```python
from build123d import *

# Parameters (mm, degrees)
SKETCH_1_W          = 10
SKETCH_1_H          = 5
EXTRUDE_1_DEPTH     = 0.5
SKETCH_2_W          = 3
SKETCH_2_H          = 3
EXTRUDE_2_DEPTH     = 0.5
SKETCH_3_W          = 10
SKETCH_3_H          = 5
EXTRUDE_3_DEPTH     = 0.5
EXTRUDE_4_DEPTH     = 5
CUT_EXTRUDE_3_DEPTH = 5
SKETCH_6_W          = 1.6
SKETCH_6_H          = 1.6
CUT_EXTRUDE_4_DEPTH = 1.5
SKETCH_7_W          = 10
SKETCH_7_H          = 0.5
CUT_EXTRUDE_5_DEPTH = 1
SKETCH_8_W          = 10
SKETCH_8_H          = 4
EXTRUDE_5_DEPTH     = 1
SKETCH_11_W         = 10
SKETCH_11_H         = 4
SKETCH_11_W_2       = 3
SKETCH_11_H_2       = 3
CUT_EXTRUDE_6_DEPTH = 0.5
CUT_EXTRUDE_7_REACH = 8.124
SKETCH_6_2_W        = 1.6
SKETCH_6_2_H        = 1.6
SKETCH_12_W         = 10
SKETCH_12_H         = 5
CUT_EXTRUDE_8_DEPTH = 6.937171044
SKETCH_13_W         = 3
SKETCH_13_H         = 3
EXTRUDE_6_DEPTH     = 3
SKETCH_14_W         = 1.7
SKETCH_14_H         = 1.7
CUT_EXTRUDE_9_DEPTH = 4


with BuildPart() as part:
    # 草图1 → 凸台-拉伸1 (new body)
    with BuildSketch(Plane(origin=(0, 0, 0), x_dir=(1, 0, 0), z_dir=(0, 1, 0))):
        Rectangle(SKETCH_1_W, SKETCH_1_H)
    extrude(amount=EXTRUDE_1_DEPTH)

    # 草图2 → 凸台-拉伸2 (add)
    with BuildSketch(Plane(origin=(0, 0.5, 0), x_dir=(1, 0, 0), z_dir=(0, 1, 0))):
        Rectangle(SKETCH_2_W, SKETCH_2_H)
    extrude(amount=EXTRUDE_2_DEPTH)

    # 草图3 → 凸台-拉伸3 (add)
    with BuildSketch(Plane(origin=(0, 1, 0), x_dir=(1, 0, 0), z_dir=(0, 1, 0))):
        Rectangle(SKETCH_3_W, SKETCH_3_H)
    extrude(amount=EXTRUDE_3_DEPTH)

    # 草图4 → 凸台-拉伸4 (add)
    with BuildSketch(Plane.XY.offset(2.5)):
        with BuildLine():
            Line((-5, 1.5), (5, 1.5))
            ThreePointArc((5, 1.5), (0, 2.5), (-5, 1.5))
        make_face()
    extrude(amount=-EXTRUDE_4_DEPTH)

    # 草图5 → 切除-拉伸3 (cut)
    with BuildSketch(Plane.XY.offset(2.5)):
        with BuildLine():
            Line((-4.75, 2.75), (-4.25, 2.75))
            Line((-4.25, 2.75), (-4.25, 1.535662375))
            ThreePointArc((-4.25, 1.535662375), (-4.50094573, 1.445961936), (-4.75, 1.35113631))
            Line((-4.75, 1.35113631), (-4.75, 2.75))
        make_face()
        with BuildLine():
            Line((-3.75, 2.75), (-3.75, 1.697389285))
            ThreePointArc((-3.75, 1.697389285), (-3.500697998, 1.769788877), (-3.25, 1.837195875))
            Line((-3.25, 1.837195875), (-3.25, 2.75))
            Line((-3.25, 2.75), (-3.75, 2.75))
        make_face()
        with BuildLine():
            Line((-2.75, 2.75), (-2.75, 1.95580576))
            ThreePointArc((-2.75, 1.95580576), (-2.500480176, 2.007256715), (-2.25, 2.053808027))
            Line((-2.25, 2.053808027), (-2.25, 2.75))
            Line((-2.25, 2.75), (-2.75, 2.75))
        make_face()
        with BuildLine():
            Line((-1.75, 2.75), (-1.75, 2.131673028))
            ThreePointArc((-1.75, 2.131673028), (-1.50028119, 2.163138904), (-1.25, 2.189764295))
            Line((-1.25, 2.189764295), (-1.25, 2.75))
            Line((-1.25, 2.75), (-1.75, 2.75))
        make_face()
        with BuildLine():
            Line((-0.75, 2.75), (-0.75, 2.228347352))
            ThreePointArc((-0.75, 2.228347352), (-0.500092618, 2.240377492), (-0.25, 2.247595932))
            Line((-0.25, 2.247595932), (-0.25, 2.75))
            Line((-0.25, 2.75), (-0.75, 2.75))
        make_face()
        with BuildLine():
            Line((0.25, 2.75), (0.25, 2.247595932))
            ThreePointArc((0.25, 2.247595932), (0.500092618, 2.240377492), (0.75, 2.228347352))
            Line((0.75, 2.228347352), (0.75, 2.75))
            Line((0.75, 2.75), (0.25, 2.75))
        make_face()
        with BuildLine():
            Line((1.25, 2.75), (1.25, 2.189764295))
            ThreePointArc((1.25, 2.189764295), (1.50028119, 2.163138904), (1.75, 2.131673028))
            Line((1.75, 2.131673028), (1.75, 2.75))
            Line((1.75, 2.75), (1.25, 2.75))
        make_face()
        with BuildLine():
            Line((2.25, 2.75), (2.25, 2.053808027))
            ThreePointArc((2.25, 2.053808027), (2.500480176, 2.007256715), (2.75, 1.95580576))
            Line((2.75, 1.95580576), (2.75, 2.75))
            Line((2.75, 2.75), (2.25, 2.75))
        make_face()
        with BuildLine():
            Line((3.25, 2.75), (3.25, 1.837195875))
            ThreePointArc((3.25, 1.837195875), (3.500697998, 1.769788877), (3.75, 1.697389285))
            Line((3.75, 1.697389285), (3.75, 2.75))
            Line((3.75, 2.75), (3.25, 2.75))
        make_face()
        with BuildLine():
            Line((4.25, 2.75), (4.25, 1.535662375))
            ThreePointArc((4.25, 1.535662375), (4.50094573, 1.445961936), (4.75, 1.35113631))
            Line((4.75, 1.35113631), (4.75, 2.75))
            Line((4.75, 2.75), (4.25, 2.75))
        make_face()
    extrude(amount=-CUT_EXTRUDE_3_DEPTH, mode=Mode.SUBTRACT)

    # 草图6 → 切除-拉伸4 (cut)
    with BuildSketch(Plane.XZ):
        Rectangle(SKETCH_6_W, SKETCH_6_H)
    extrude(amount=-CUT_EXTRUDE_4_DEPTH, mode=Mode.SUBTRACT)

    # 草图7 → 切除-拉伸5 (cut)
    with BuildSketch(Plane.XZ):
        with Locations((0, 2.25)):
            Rectangle(SKETCH_7_W, SKETCH_7_H)
        with Locations((0, -2.25)):
            Rectangle(SKETCH_7_W, SKETCH_7_H)
    extrude(amount=-CUT_EXTRUDE_5_DEPTH, mode=Mode.SUBTRACT)

    # 草图8 → 凸台-拉伸5 (add)
    with BuildSketch(Plane.XZ):
        Rectangle(SKETCH_8_W, SKETCH_8_H)
    extrude(amount=EXTRUDE_5_DEPTH)

    # 草图11 → 切除-拉伸6 (cut)
    with BuildSketch(Plane(origin=(0, 0.5, 0), x_dir=(1, 0, 0), z_dir=(0, 1, 0))):
        Rectangle(SKETCH_11_W, SKETCH_11_H)
        Rectangle(SKETCH_11_W_2, SKETCH_11_H_2, mode=Mode.SUBTRACT)
    extrude(amount=-CUT_EXTRUDE_6_DEPTH, mode=Mode.SUBTRACT)

    # 草图6<2> → 切除-拉伸7 (cut, up to next)
    with BuildSketch(Plane.XZ, mode=Mode.PRIVATE) as cut_extrude_7_sk1:
        Rectangle(SKETCH_6_2_W, SKETCH_6_2_H)
    cut_extrude_7_tool1 = extrude(cut_extrude_7_sk1.sketch, amount=CUT_EXTRUDE_7_REACH, mode=Mode.PRIVATE) & part.part
    add(cut_extrude_7_tool1.solids().sort_by_distance((0, 0, 0))[0], mode=Mode.SUBTRACT)

    # 草图12 → 切除-拉伸8 (cut, through all)
    with BuildSketch(Plane.XZ.offset(-1)):
        Rectangle(SKETCH_12_W, SKETCH_12_H)
    extrude(amount=-CUT_EXTRUDE_8_DEPTH, mode=Mode.SUBTRACT)

    # 草图13 → 凸台-拉伸6 (add)
    with BuildSketch(Plane(origin=(0, 1, 0), x_dir=(1, 0, 0), z_dir=(0, 1, 0))):
        Rectangle(SKETCH_13_W, SKETCH_13_H)
    extrude(amount=EXTRUDE_6_DEPTH)

    # 草图14 → 切除-拉伸9 (cut)
    with BuildSketch(Plane.XZ.offset(1)):
        Rectangle(SKETCH_14_W, SKETCH_14_H)
    extrude(amount=-CUT_EXTRUDE_9_DEPTH, mode=Mode.SUBTRACT)


solid = part.part
```
Input: part model. Units: mm. Frame: model coordinates. A direction names the side the tool comes from. Round coordinates to 2 decimals unless told otherwise and drop trailing zeros. Order: outer loops, then holes, each group sorted by start corner. A loop starts at its lowest first (then second) coordinate and runs counter-clockwise, first axis right, second up. Notation, with made-up numbers: (88, -25.5) - (96, -25.5) arc R24 ccw to (96, 8.5) - close; hole circle Ø2 at (21, 64.5). An arc over 180 degrees is marked (long way). One line per question, with ' | ' between items. Start each with the question number.
1) Cut plane D-D, the plane z = -0.95. Return the cut outline in (x, y).
2) Set-up query: faces 1 (the flat face through (1.5, 2, 0)), 2 (the flat face through (0, -1, 1)), 3 (the flat face through (0, 2, 1.5)), 4 (the flat face through (0.85, 1, 0)). Return all of +Z, -Z, +X, -X, +Y, -Y with unobstructed straight access to the full face (end or side cutting, diameter ignored); none if empty.
3) Contact query for flat-ended pins moving along their axis: P1, Ø1.5, axis at y = 1.5, z = 0, coming from the -X side; P2, Ø1.4, axis at x = -0.5, y = 1, coming from the -Z side; P3, Ø0.5, axis at y = 0.5, z = 0.5, coming from the +X side; P4, Ø1.5, axis at x = 3, y = 1, coming from the -Z side. Output: stop coordinate, or through.
4) Cut plane C-C, the plane x = 0.5. Return the cut outline in (y, z), then the cut area to 3 significant figures.
5) Ray query, probe 1 along Z at (x, y) = (0.25, 1.75); probe 2 along Y at (x, z) = (-3.25, 1.3). Return the intervals inside material, ascending.
6) Cut plane B-B, the plane z = 0.4. Return the cut outline in (x, y), then the cut area to 3 significant figures.
7) Pull-direction query (Z, two-part tool) for faces 5 (the flat face through (-1.5, 2, 0)), 6 (the flat face through (0, 1, 0.85)), 7 (the flat face through (0, 2, -1.5)); classes: +Z half, -Z half, draft (parallel to the pull), parting line (faces both ways), or undercut.
8) Cut plane A-A, the plane y = 1.9. Return the cut outline in (x, z).
Worked out:
1) outline: (-5, -1) - (5, -1) - (5, 0) - (1.5, 0) - (1.5, 4) - (-1.5, 4) - (-1.5, 0) - (-5, 0) - close
2) face 1: +Z, -Z, +X, +Y | face 2: +Z, -Z, +X, -X, -Y | face 3: +Z, +X, -X, +Y | face 4: -Y
3) P1: stops at x = -1.5 | P2: stops at z = -1.5 | P3: stops at x = 1.5 | P4: passes through
4) outline: (-1, -2) - (0, -2) - (0, -1.5) - (4, -1.5) - (4, 1.5) - (0, 1.5) - (0, 2) - (-1, 2) - (-1, 0.85) - (3, 0.85) - (3, -0.85) - (-1, -0.85) - close | area: 9.20 mm^2
5) probe 1: z = -1.5 to -0.85, 0.85 to 1.5 | probe 2: y = -1 to 0
6) outline: (-5, -1) - (-0.85, -1) - (-0.85, 3) - (0.85, 3) - (0.85, -1) - (5, -1) - (5, 0) - (1.5, 0) - (1.5, 4) - (-1.5, 4) - (-1.5, 0) - (-5, 0) - close | area: 15.2 mm^2
7) face 5: draft | face 6: undercut | face 7: -Z half
8) outline: (-1.5, -1.5) - (1.5, -1.5) - (1.5, 1.5) - (-1.5, 1.5) - close; hole (-0.85, -0.85) - (0.85, -0.85) - (0.85, 0.85) - (-0.85, 0.85) - close
